Design review of the part built by this model. Coordinates are the model's own, in mm. Give positions to 0.01 mm unless a question says otherwise; leave off trailing zeros. Loops run counter-clockwise (first coordinate to the right, second up) from the corner with the lowest first, then second, coordinate; pieces in that order, holes last. Notation, with made-up numbers: (11.5, -30) - (57.5, -30) arc R21 ccw to (57.5, -17) - close; hole circle Ø4 at (13, 31). An arc over 180 degrees is marked (long way). One line per item, written item: value. Start each with the question number.
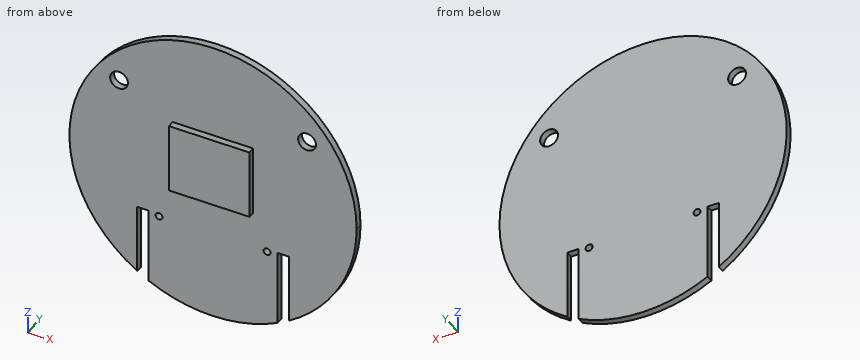
```python
from build123d import *

# Parameters (mm, degrees)
F0_R     = 1.5
F0_R_2   = 3.875
F0_W     = 35
F0_H     = 30
F1_DEPTH = 3
F2_DEPTH = 6


with BuildPart() as f1:
    # F0 (on Front) → F1 (new body)
    with BuildSketch(Plane.XZ):
        with BuildLine():
            ThreePointArc((33, -53.077773), (54.629433, -30.362395), (62.5, 0))
            ThreePointArc((62.5, 0), (-30.362395, 54.629433), (-33, -53.077773))
            Line((-33, -53.077773), (-33, -23.207187))
            Line((-33, -23.207187), (-28, -23.207187))
            Line((-28, -23.207187), (-28, -55.877097))
            ThreePointArc((-28, -55.877097), (0, -62.5), (28, -55.877097))
            Line((28, -55.877097), (28, -23.207187))
            Line((28, -23.207187), (33, -23.207187))
            Line((33, -23.207187), (33, -53.077773))
        make_face()
        with Locations((-23.5, -24.207187)):
            Circle(F0_R, mode=Mode.SUBTRACT)
        with Locations((23.5, -24.207187)):
            Circle(F0_R, mode=Mode.SUBTRACT)
        with Locations((-40.913567, 33.097895)):
            Circle(F0_R_2, mode=Mode.SUBTRACT)
        with Locations((0, 6.792813)):
            Rectangle(F0_W, F0_H, mode=Mode.SUBTRACT)
        with Locations((40.913567, 33.097895)):
            Circle(F0_R_2, mode=Mode.SUBTRACT)
        with Locations((0, 6.792813)):
            Rectangle(F0_W, F0_H)
    extrude(amount=F1_DEPTH)

    # F0 (on Front) → F2 (join)
    with BuildSketch(Plane.XZ):
        with Locations((0, 6.792813)):
            Rectangle(F0_W, F0_H)
    extrude(amount=F2_DEPTH)


solid = f1.part
```
(1) Take a section at C-C on x = 23.5. State the section outline as (y, z) points.
(2) Take a section at A-A on x = 0. State the section outline as (y, z) points, and give its area (3 significant figures).
(3) For pin 1 Ø3.5 at (x, y) = (-5, -5) entering from +Z; pin 2 Ø3 at (y, z) = (-3, 44.5) entering from +X; pin 3 Ø0.9 at (y, z) = (-4.5, 12) entering from +X, all flat-tipped, find the tip position at first contact; note any pin that passes through.
(4) Take a section at B-B on z = 12.5. State the section outline as (x, y) points, and give its area (3 significant figures).
(5) Take a section at D-D on y = -4.8. State the section outline as (x, z) points.
(6) To check wall thickness, follow L1, parallel to X at y = -2.5, z = -35.5; L2, parallel to Y at x = 4, z = 49.5; L3, parallel to Z at x = -13, y = -4.4. State the ranges of each line that lie inside material, in increasing order. Write a range as from..to.
Here are the results:
1. outline: (-3, -57.91) - (0, -57.91) - (0, -25.71) - (-3, -25.71) - close; (-3, -22.71) - (0, -22.71) - (0, 57.91) - (-3, 57.91) - close
2. outline: (-6, -8.21) - (-3, -8.21) - (-3, -62.5) - (0, -62.5) - (0, 62.5) - (-3, 62.5) - (-3, 21.79) - (-6, 21.79) - close
2. area: 465 mm²
3. pin 1: z = 21.79
3. pin 2: x = 45.36
3. pin 3: x = 17.5
4. outline: (-61.24, -3) - (-17.5, -3) - (-17.5, -6) - (17.5, -6) - (17.5, -3) - (61.24, -3) - (61.24, 0) - (-61.24, 0) - close
4. area: 472 mm²
5. outline: (-17.5, -8.21) - (17.5, -8.21) - (17.5, 21.79) - (-17.5, 21.79) - close
6. L1: -51.44..-33, -28..28, 33..51.44
6. L2: -3..0
6. L3: -8.21..21.79
